```python
from build123d import *

# Parameters (mm, degrees)
BOSS_EXTRUDE1_DEPTH = 191
SKETCH2_W           = 3
SKETCH2_H           = 1
SKETCH2_W_2         = 1
SKETCH2_H_2         = 4
CUT_EXTRUDE1_DEPTH  = 193.59023859
FILLET1_R           = 0.25


with BuildPart() as part:
    # Sketch1 → Boss-Extrude1 (new body)
    with BuildSketch(Plane.XY):
        with BuildLine():
            Line((0, 3), (-15, 3))
            ThreePointArc((-15, 3), (-19.242640687, 1.242640687), (-21, -3))
            Line((-21, -3), (-21, -7))
            ThreePointArc((-21, -7), (-19.242640687, -11.242640687), (-15, -13))
            Line((-15, -13), (0, -13))
            ThreePointArc((0, -13), (4.242640687, -11.242640687), (6, -7))
            Line((6, -7), (6, -3))
            ThreePointArc((6, -3), (4.242640687, 1.242640687), (0, 3))
        make_face()
        with BuildLine():
            Line((0, 0), (-15, 0))
            ThreePointArc((-15, 0), (-17.121320344, -0.878679656), (-18, -3))
            Line((-18, -3), (-18, -7))
            ThreePointArc((-18, -7), (-17.121320344, -9.121320344), (-15, -10))
            Line((-15, -10), (0, -10))
            ThreePointArc((0, -10), (2.121320344, -9.121320344), (3, -7))
            Line((3, -7), (3, -3))
            ThreePointArc((3, -3), (2.121320344, -0.878679656), (0, 0))
        make_face(mode=Mode.SUBTRACT)
    extrude(amount=BOSS_EXTRUDE1_DEPTH)

    # Sketch2 → Cut-Extrude1 (cut, through all)
    with BuildSketch(Plane.XY.offset(191)):
        with Locations((-7.5, 3)):
            Rectangle(SKETCH2_W, SKETCH2_H)
        with Locations((-12.5, 3)):
            Rectangle(SKETCH2_W, SKETCH2_H)
        with Locations((-2.5, 3)):
            Rectangle(SKETCH2_W, SKETCH2_H)
        with Locations((-2.5, -13)):
            Rectangle(SKETCH2_W, SKETCH2_H)
        with Locations((-12.5, -13)):
            Rectangle(SKETCH2_W, SKETCH2_H)
        with Locations((-7.5, -13)):
            Rectangle(SKETCH2_W, SKETCH2_H)
        with Locations((6, -5)):
            Rectangle(SKETCH2_W_2, SKETCH2_H_2)
        with Locations((-21, -5)):
            Rectangle(SKETCH2_W_2, SKETCH2_H_2)
    extrude(amount=-CUT_EXTRUDE1_DEPTH, mode=Mode.SUBTRACT)

    # Fillet1
    fillet1_edges = [part.edges().sort_by_distance(p)[0] for p in [
        (-20.5, -7, 95.5),
        (-20.5, -3, 95.5),
        (-14, -13, 95.5),
        (-11, -12.5, 95.5),
        (-6, -12.5, 95.5),
        (-11, -13, 95.5),
        (-9, -13, 95.5),
        (-6, -13, 95.5),
        (-4, -13, 95.5),
        (-14, -12.5, 95.5),
        (-9, -12.5, 95.5),
        (-1, -13, 95.5),
        (-1, -12.5, 95.5),
        (5.5, -7, 95.5),
        (-4, -12.5, 95.5),
        (5.5, -3, 95.5),
        (-1, 3, 95.5),
        (-4, 3, 95.5),
        (-6, 3, 95.5),
        (-14, 3, 95.5),
        (-11, 3, 95.5),
        (-9, 3, 95.5),
        (-1, 2.5, 95.5),
        (-4, 2.5, 95.5),
        (-6, 2.5, 95.5),
        (-9, 2.5, 95.5),
        (-11, 2.5, 95.5),
        (-14, 2.5, 95.5),
    ]]
    fillet(fillet1_edges, radius=FILLET1_R - 0.0001)  # a hair under: the kernel refuses the full size


solid = part.part
```
Check sheet for the modelled part. Datum: model origin and axes. Units: mm. A direction names the side the tool comes from. Coordinates: 2 decimals unless noted, no trailing zeros. Write item = value, one per line. Start each with the question number.
1) Mould release check, pull along Y, two halves, no side actions. Record for faces 1 (the cylindrical face through (-17.1, -0.86, 94.16)), 2 (the flat face through (-7.7, 0.4, 0)), 3 (the cylindrical face through (-19.289, -11.196, 94.163)), 4 (the cylindrical face through (-19.196, 1.289, 94.163)): +Y half, -Y half, draft (parallel to the pull), parting line (faces both ways), or undercut.
2) Go/stop test with flat-tipped pins: P1, Ø1, axis at y = -0.5, z = 118.5, coming from the -X side; P2, Ø1.8, axis at y = -5.5, z = 125.5, coming from the -X side; P3, Ø1.3, axis at x = -12.5, z = 62, coming from the -Y side. Record where each tip stops, or that it passes through.
3) Access from +Z, -Z, +X, -X, +Y, -Y to the whole of each face (thin tool, end or side, straight path). Record for faces 5 (the flat face through (-7, 0, 94)), 6 (the cylindrical face through (4.196, -11.289, 94.163)), 7 (the flat face through (5.5, -5, 97)), 8 (the flat face through (-20.5, -5, 97)).
4) Material ranges on L1, parallel to Y at x = -3.25, z = 27; L2, parallel to X at y = -2.75, z = 155; L3, parallel to Y at x = -15.25, z = 133.5, recorded low to high.
Ans:
q1.face_1 = undercut
q1.face_2 = draft
q1.face_3 = -Y half
q1.face_4 = +Y half
q2.P1 = -20.66
q2.P2 = -20.5
q2.P3 = -12.5
q3.face_5 = +Z, -Z
q3.face_6 = +Z, -Z, +X, -Y
q3.face_7 = +Z, -Z, +X
q3.face_8 = +Z, -Z, -X
q4.L1 = -12.5 to -10, 0 to 2.5
q4.L2 = -20.99 to -17.99, 2.99 to 5.99
q4.L3 = -12.99 to -9.99, -0.01 to 2.99
